Verification items for the finished model (mm, model axes). A direction names the side the tool comes from. Give positions to 0.01 mm unless a question says otherwise; leave off trailing zeros. Write each loop counter-clockwise with the first axis right and the second up, starting at its lowest first coordinate (ties: lowest second). Pieces come first, ordered by that corner, then holes. Notation, with made-up numbers: (15.25, 50) -> (52.25, 50) arc R30 ccw to (52.25, 77) -> close; hole circle Ø2 at (88.5, 2). An arc over 180 degrees is marked (long way). Use one line per item in the form item = value. Start each with the question number.
(1) Section check C-C, the plane z = -10.5. Record the cut outline in (x, y).
(2) Section check B-B, the plane y = 0. Record the cut outline in (x, z), plus the area to 3 significant figures.
(3) Set-up check for faces 4 (the face through (-13, 26, -12.5)), 5 (the face through (-47, 42, 17.5)), 6 (the face through (3.755, 11.923, 0.315)): record each of +Z, -Z, +X, -X, +Y, -Y from which the full face is reachable in a straight line by a thin tool's end or side.
(4) Release check for a two-part mould opening along X. For faces 1 (the face through (7.56, 24.005, 21.874)), 2 (the face through (-47, -42, -17.5)), 3 (the face through (-42.898, -55.946, -0.245)) record: pulls with the +X half, pulls with the -X half, needs draft (parallel to the pull), parting line crosses it, or undercut.
(5) Section check D-D, the plane z = 19.5. Record the cut outline in (x, y).
(6) Section check A-A, the plane x = 0. State how many separate pieces and enclosed holes the cut face has, plus the area to 3 significant figures.
(7) Scan lines: L1, parallel to Y at x = -38.5, z = 1.5; L2, parallel to X at y = 0, z = 9; L3, parallel to X at y = 16.5, z = -14. Record each from-to range of solid material in increasing order.
(8) Depth check by flat-ended pin: pin 1 Ø10.5 at (x, y) = (-38.47, 22.21) entering from +Z; pin 2 Ø13 at (x, y) = (38.47, 22.21) entering from -Z; pin 3 Ø12 at (x, z) = (-15, -4.5) entering from +Y; pin 4 Ø5 at (x, y) = (-38.47, -22.21) entering from -Z. Enter the tip coordinate at first touch or a pass-through.
from build123d import *

# Parameters (mm, degrees)
CUT_EXTRUDE2_REACH = 37
SKETCH9_R          = 4


with BuildPart() as part:
    # Sketch8 → Revolve3 (revolve)
    with BuildSketch(Plane(origin=(0, 0, 0), x_dir=(0, 0, -1), z_dir=(1, 0, 0))):
        Polygon((22.5, 12.5), (-22.5, 12.5), (-22.5, 25), (-12.5, 27.679491924), (-12.5, 61.160254038), (-17.5, 62.5), (-17.5, 70.5), (17.5, 70.5), (17.5, 62.5), (12.5, 61.160254038), (12.5, 27.679491924), (22.5, 25), align=None)
    revolve(axis=Axis((0, 0, 62.265479925), (0, 0, -1)))

    # Sketch9 → Cut-Extrude2 (cut, up to next)
    with BuildSketch(Plane.XY.offset(12.5), mode=Mode.PRIVATE) as cut_extrude2_sk1:
        with Locations((0, 44.419872981)):
            Circle(SKETCH9_R)
    cut_extrude2_tool1 = extrude(cut_extrude2_sk1.sketch, amount=-CUT_EXTRUDE2_REACH, mode=Mode.PRIVATE) & part.part
    add(cut_extrude2_tool1.solids().sort_by_distance((0, 44.419873, 12.5))[0], mode=Mode.SUBTRACT)
    # Sketch9 → Cut-Extrude2 (cut, up to next)
    with BuildSketch(Plane.XY.offset(12.5), mode=Mode.PRIVATE) as cut_extrude2_sk2:
        with Locations((38.468738434, 22.209936491)):
            Circle(SKETCH9_R)
    cut_extrude2_tool2 = extrude(cut_extrude2_sk2.sketch, amount=-CUT_EXTRUDE2_REACH, mode=Mode.PRIVATE) & part.part
    add(cut_extrude2_tool2.solids().sort_by_distance((38.468738, 22.209936, 12.5))[0], mode=Mode.SUBTRACT)
    # Sketch9 → Cut-Extrude2 (cut, up to next)
    with BuildSketch(Plane.XY.offset(12.5), mode=Mode.PRIVATE) as cut_extrude2_sk3:
        with Locations((38.468738434, -22.209936491)):
            Circle(SKETCH9_R)
    cut_extrude2_tool3 = extrude(cut_extrude2_sk3.sketch, amount=-CUT_EXTRUDE2_REACH, mode=Mode.PRIVATE) & part.part
    add(cut_extrude2_tool3.solids().sort_by_distance((38.468738, -22.209936, 12.5))[0], mode=Mode.SUBTRACT)
    # Sketch9 → Cut-Extrude2 (cut, up to next)
    with BuildSketch(Plane.XY.offset(12.5), mode=Mode.PRIVATE) as cut_extrude2_sk4:
        with Locations((0, -44.419872981)):
            Circle(SKETCH9_R)
    cut_extrude2_tool4 = extrude(cut_extrude2_sk4.sketch, amount=-CUT_EXTRUDE2_REACH, mode=Mode.PRIVATE) & part.part
    add(cut_extrude2_tool4.solids().sort_by_distance((0, -44.419873, 12.5))[0], mode=Mode.SUBTRACT)
    # Sketch9 → Cut-Extrude2 (cut, up to next)
    with BuildSketch(Plane.XY.offset(12.5), mode=Mode.PRIVATE) as cut_extrude2_sk5:
        with Locations((-38.468738434, -22.209936491)):
            Circle(SKETCH9_R)
    cut_extrude2_tool5 = extrude(cut_extrude2_sk5.sketch, amount=-CUT_EXTRUDE2_REACH, mode=Mode.PRIVATE) & part.part
    add(cut_extrude2_tool5.solids().sort_by_distance((-38.468738, -22.209936, 12.5))[0], mode=Mode.SUBTRACT)
    # Sketch9 → Cut-Extrude2 (cut, up to next)
    with BuildSketch(Plane.XY.offset(12.5), mode=Mode.PRIVATE) as cut_extrude2_sk6:
        with Locations((-38.468738434, 22.209936491)):
            Circle(SKETCH9_R)
    cut_extrude2_tool6 = extrude(cut_extrude2_sk6.sketch, amount=-CUT_EXTRUDE2_REACH, mode=Mode.PRIVATE) & part.part
    add(cut_extrude2_tool6.solids().sort_by_distance((-38.468738, 22.209936, 12.5))[0], mode=Mode.SUBTRACT)


solid = part.part
Completed:
q1.outline = circle Ø141 at (0, 0); hole circle Ø8 at (-38.47, -22.21); hole circle Ø8 at (-38.47, 22.21); hole circle Ø25 at (0, 0); hole circle Ø8 at (0, -44.42); hole circle Ø8 at (0, 44.42); hole circle Ø8 at (38.47, -22.21); hole circle Ø8 at (38.47, 22.21)
q2.outline = (-70.5, -17.5) -> (-62.5, -17.5) -> (-61.16, -12.5) -> (-27.68, -12.5) -> (-25, -22.5) -> (-12.5, -22.5) -> (-12.5, 22.5) -> (-25, 22.5) -> (-27.68, 12.5) -> (-61.16, 12.5) -> (-62.5, 17.5) -> (-70.5, 17.5) -> close; (12.5, -22.5) -> (25, -22.5) -> (27.68, -12.5) -> (61.16, -12.5) -> (62.5, -17.5) -> (70.5, -17.5) -> (70.5, 17.5) -> (62.5, 17.5) -> (61.16, 12.5) -> (27.68, 12.5) -> (25, 22.5) -> (12.5, 22.5) -> close
q2.area = 3,630 mm²
q3.face_4 = -Z
q3.face_5 = +Z
q3.face_6 = +Z, -Z
q4.face_1 = undercut
q4.face_2 = needs draft
q4.face_3 = parting line crosses it
q5.outline = circle Ø51.61 at (0, 0); hole circle Ø25 at (0, 0)
q6.separate_pieces = 4
q6.enclosed_holes = 0
q6.area = 3,230 mm²
q7.L1 = -59.06 to -26.21, -18.21 to 18.21, 26.21 to 59.06
q7.L2 = -70.5 to -12.5, 12.5 to 70.5
q7.L3 = -68.54 to -59.31, -21.72 to 21.72, 59.31 to 68.54
q8.pin_1 = 12.5
q8.pin_2 = -12.5
q8.pin_3 = 69.92
q8.pin_4 = through
